The drawing under review shows one solid part. Ordinate dimensions are in mm from its lowest x, y, z. Coordinates: 2 decimals unless noted, no trailing zeros. Order: outer loops, then holes, each group sorted by start corner. A loop starts at its lowest first (then second) coordinate and runs counter-clockwise, first axis right, second up.
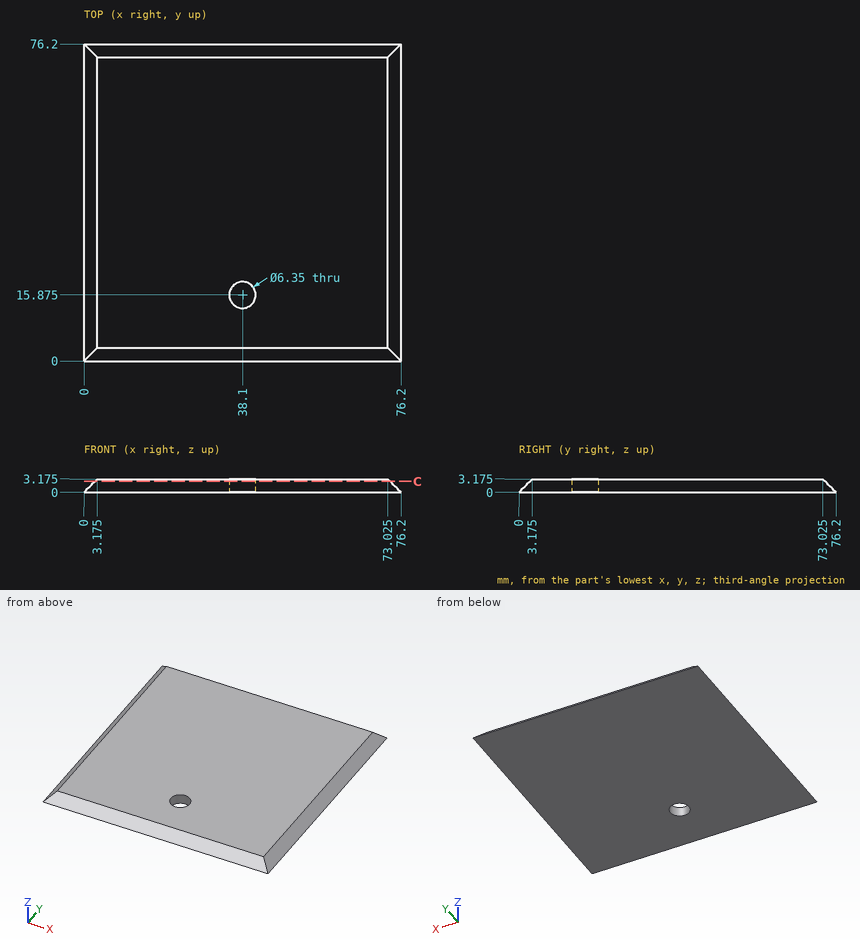
1. Insertion check: pin 1 (5 mm diameter, centred on x = 53.5, y = 26.5, fed in from -Z); pin 2 (1.5 mm diameter, centred on y = 62, z = 2.5, fed in from +X). Each pin has a flat end and moves straight along its axis. Give the tip position at first contact, or say it passes through.
2. To check wall thickness, follow line 1 (Y direction, x = 38.1, z = 0.85); line 2 (Y direction, x = 38.1, z = 0.6); line 3 (X direction, y = 67, z = 1.5). State the ranges of each line that lie inside material, in increasing order.
3. Add section C-C (z = 2.6). Give the boundary of the cut face in (x, y) (3 decimals), and give its area (3 significant figures).
Solution:
1. pin 1: stops at z = 0
1. pin 2: stops at x = 74.45
2. line 1: y = 0.85 to 12.7, 19.05 to 75.35
2. line 2: y = 0.6 to 12.7, 19.05 to 75.6
2. line 3: x = 1.5 to 74.7
3. outline: (2.6, 2.6) - (73.6, 2.6) - (73.6, 73.6) - (2.6, 73.6) - close; hole circle Ø6.35 at (38.1, 15.875)
3. area: 5,010 mm2
